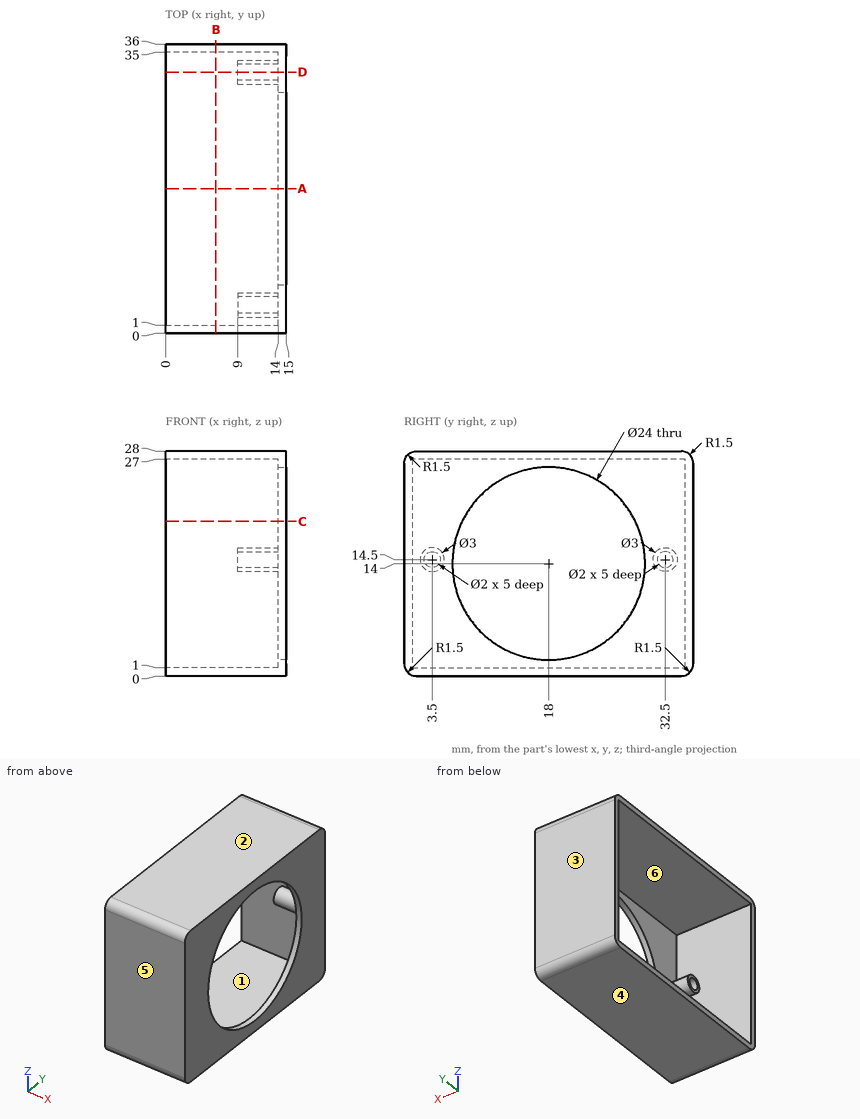
Source: three-view drawing plus pictorial views. Frame: mm from the lowest corner of the part. A direction names the side the tool comes from. Round coordinates to 2 decimals unless told otherwise and drop trailing zeros. Loops run counter-clockwise (first coordinate to the right, second up) from the corner with the lowest first, then second, coordinate; pieces in that order, holes last.
Q1. Section D-D on y = 32.5. Return loops of the section in (x, z), plus the area to 3 significant figures.
Q2. Section B-B on x = 6.25. Return loops of the section in (y, z), plus the area to 3 significant figures.
Q3. Access query for the marked faces 1 and 2. Directions: +Z, -Z, +X, -X, +Y, -Y. A direction counts if a zero-diameter tool reaches every point of the face in a straight line with its end or side. Return the directions, or none.
Q4. Pin query (flat end, axial travel): P1, Ø2, axis at y = 11.5, z = 24, coming from the -X side; P2, Ø1.5, axis at y = 32, z = 14, coming from the -X side. Return the tip coordinate at first contact, or that it passes through.
Q5. Section C-C on z = 19.25. Return loops of the section in (x, y).
Q6. Material intervals for L1, parallel to Y at x = 11.6, z = 14.5; L2, parallel to Z at x = 10.85, y = 32.5; L3, parallel to Z at x = 4.5, y = 18, sorted ascending.
Q7. Section A-A on y = 18. Return loops of the section in (x, z), plus the area to 3 significant figures.
Q8. Pull-direction query (Y, two-part tool) for the marked faces 3, 4, 5 and 6; classes: released by +Y, released by -Y, zero draft, split by the parting line, or undercut.
Evaluation:
1. outline: (0, 0) - (15, 0) - (15, 28) - (0, 28) - (0, 27) - (14, 27) - (14, 16) - (9, 16) - (9, 15.5) - (14, 15.5) - (14, 13.5) - (9, 13.5) - (9, 13) - (14, 13) - (14, 1) - (0, 1) - close
1. area: 61.0 mm2
2. outline: (0, 1.5) arc R1.5 ccw to (1.5, 0) - (34.5, 0) arc R1.5 ccw to (36, 1.5) - (36, 26.5) arc R1.5 ccw to (34.5, 28) - (1.5, 28) arc R1.5 ccw to (0, 26.5) - close; hole (1, 1) - (35, 1) - (35, 27) - (1, 27) - close
2. area: 122 mm2
3. face 1: -X
3. face 2: +Z, +X, -X, +Y, -Y
4. P1: stops at x = 14
4. P2: stops at x = 9
5. outline: (0, 0) - (15, 0) - (15, 7.21) - (14, 7.21) - (14, 1) - (0, 1) - close; (0, 35) - (14, 35) - (14, 28.79) - (15, 28.79) - (15, 36) - (0, 36) - close
6. L1: y = 0 to 1, 2 to 2.5, 4.5 to 5, 31 to 31.5, 33.5 to 34, 35 to 36
6. L2: z = 0 to 1, 13 to 13.5, 15.5 to 16, 27 to 28
6. L3: z = 0 to 1, 27 to 28
7. outline: (0, 0) - (15, 0) - (15, 2) - (14, 2) - (14, 1) - (0, 1) - close; (0, 27) - (14, 27) - (14, 26) - (15, 26) - (15, 28) - (0, 28) - close
7. area: 32.0 mm2
8. face 3: released by +Y
8. face 4: zero draft
8. face 5: released by -Y
8. face 6: undercut
